```python
from build123d import *

# Parameters (mm, degrees)
STOCK_ACRYLIC_BAY_WALL_MASTER_1_START     = 163.456714755
STOCK_ACRYLIC_BAY_WALL_MASTER_1_OUTLINE_R = 2
STOCK_ACRYLIC_BAY_WALL_MASTER_1_DEPTH     = 5
SKETCH1_W                                 = 243.769145362
SKETCH1_H                                 = 5
BOSS_EXTRUDE1_DEPTH                       = 5
SKETCH2_W                                 = 25.2
SKETCH2_H                                 = 5
CUT_EXTRUDE1_DEPTH                        = 158.991773268
SKETCH3_R                                 = 1.6
CUT_EXTRUDE2_DEPTH                        = 158.991773268
SKETCH4_R                                 = 2
SKETCH4_W                                 = 27
SKETCH4_H                                 = 46.8
CUT_EXTRUDE3_DEPTH                        = 158.991773268
SKETCH5_R                                 = 22.5
SKETCH5_R_2                               = 1.6
CUT_EXTRUDE4_DEPTH                        = 158.991773268


# Read off the part's stored shape, not the designer's step: Stock-acrylic-bay-wall-master-1
with BuildPart() as part:
    # Stock-acrylic-bay-wall-master-1 outline → Stock-acrylic-bay-wall-master-1 (new body)
    with BuildSketch(Plane(origin=(0, 0, 0), x_dir=(0.866025403784438, 0, 0.500000000000001), z_dir=(0.500000000000001, 0, -0.866025403784438)).offset(STOCK_ACRYLIC_BAY_WALL_MASTER_1_START)):
        Polygon((-121.884572681, 15), (121.884572681, 15), (121.884572681, 89.75), (62.4, 89.75), (62.4, 95), (37.6, 95), (37.6, 89.75), (12.4, 89.75), (12.4, 95), (-12.4, 95), (-12.4, 89.75), (-37.6, 89.75), (-37.6, 95), (-62.4, 95), (-62.4, 89.75), (-121.884572681, 89.75), align=None)
        with Locations((-87.134572681, 35)):
            Circle(STOCK_ACRYLIC_BAY_WALL_MASTER_1_OUTLINE_R, mode=Mode.SUBTRACT)
        with Locations((87.134572681, 35)):
            Circle(STOCK_ACRYLIC_BAY_WALL_MASTER_1_OUTLINE_R, mode=Mode.SUBTRACT)
        with Locations((-112.134572681, 75)):
            Circle(STOCK_ACRYLIC_BAY_WALL_MASTER_1_OUTLINE_R, mode=Mode.SUBTRACT)
        with Locations((112.134572681, 75)):
            Circle(STOCK_ACRYLIC_BAY_WALL_MASTER_1_OUTLINE_R, mode=Mode.SUBTRACT)
    extrude(amount=STOCK_ACRYLIC_BAY_WALL_MASTER_1_DEPTH)

    # Sketch1 → Boss-Extrude1 (add)
    with BuildSketch(Plane(origin=(84.228357378, 0, -145.887794416), x_dir=(-0.8660254037844382, 0, -0.5000000000000009), z_dir=(0.5000000000000009, 0, -0.8660254037844382))):
        with Locations((0, -12.5)):
            Rectangle(SKETCH1_W, SKETCH1_H)
    extrude(amount=-BOSS_EXTRUDE1_DEPTH)

    # Sketch2 → Cut-Extrude1 (cut, through all)
    with BuildSketch(Plane(origin=(84.228357378, 0, -145.887794416), x_dir=(-0.8660254037844382, 0, -0.5000000000000009), z_dir=(0.5000000000000009, 0, -0.8660254037844382))):
        with Locations((-50, -17.5)):
            Rectangle(SKETCH2_W, SKETCH2_H)
        with Locations((0, -17.5)):
            Rectangle(SKETCH2_W, SKETCH2_H)
        with Locations((50, -17.5)):
            Rectangle(SKETCH2_W, SKETCH2_H)
    extrude(amount=-CUT_EXTRUDE1_DEPTH, mode=Mode.SUBTRACT)

    # Sketch3 → Cut-Extrude2 (cut, through all)
    with BuildSketch(Plane(origin=(84.228357378, 0, -145.887794416), x_dir=(-0.8660254037844382, 0, -0.5000000000000009), z_dir=(0.5000000000000009, 0, -0.8660254037844382))):
        with Locations((13.5, -40)):
            Circle(SKETCH3_R)
        with Locations((-13.5, -40)):
            Circle(SKETCH3_R)
        with Locations((15, -69.75)):
            Circle(SKETCH3_R)
        with Locations((-15, -69.75)):
            Circle(SKETCH3_R)
        with BuildLine():
            Line((10, -47), (10, -33))
            ThreePointArc((10, -33), (9.121320344, -30.878679656), (7, -30))
            Line((7, -30), (-7, -30))
            ThreePointArc((-7, -30), (-9.121320344, -30.878679656), (-10, -33))
            Line((-10, -33), (-10, -47))
            ThreePointArc((-10, -47), (-9.121320344, -49.121320344), (-7, -50))
            Line((-7, -50), (7, -50))
            ThreePointArc((7, -50), (9.121320344, -49.121320344), (10, -47))
        make_face()
        with BuildLine():
            Line((-6, -61.5), (6, -61.5))
            ThreePointArc((6, -61.5), (8.121320344, -62.378679656), (9, -64.5))
            Line((9, -64.5), (9, -75))
            ThreePointArc((9, -75), (8.121320344, -77.121320344), (6, -78))
            Line((6, -78), (-6, -78))
            ThreePointArc((-6, -78), (-8.121320344, -77.121320344), (-9, -75))
            Line((-9, -75), (-9, -64.5))
            ThreePointArc((-9, -64.5), (-8.121320344, -62.378679656), (-6, -61.5))
        make_face()
    extrude(amount=-CUT_EXTRUDE2_DEPTH, mode=Mode.SUBTRACT)

    # Sketch4 → Cut-Extrude3 (cut, through all)
    with BuildSketch(Plane(origin=(84.228357378, 0, -145.887794416), x_dir=(-0.8660254037844382, 0, -0.5000000000000009), z_dir=(0.5000000000000009, 0, -0.8660254037844382))):
        with Locations((69.1, -54.875)):
            Circle(SKETCH4_R)
        with Locations((30.9, -54.875)):
            Circle(SKETCH4_R)
        with Locations((50, -54.875)):
            Rectangle(SKETCH4_W, SKETCH4_H)
    extrude(amount=-CUT_EXTRUDE3_DEPTH, mode=Mode.SUBTRACT)

    # Sketch5 → Cut-Extrude4 (cut, through all)
    with BuildSketch(Plane(origin=(84.228357378, 0, -145.887794416), x_dir=(-0.8660254037844382, 0, -0.5000000000000009), z_dir=(0.5000000000000009, 0, -0.8660254037844382))):
        with Locations((-51.4, -54.875)):
            Circle(SKETCH5_R)
        with Locations((-71.4, -34.875)):
            Circle(SKETCH5_R_2)
        with Locations((-31.4, -34.875)):
            Circle(SKETCH5_R_2)
        with Locations((-31.4, -74.875)):
            Circle(SKETCH5_R_2)
        with Locations((-71.4, -74.875)):
            Circle(SKETCH5_R_2)
    extrude(amount=-CUT_EXTRUDE4_DEPTH, mode=Mode.SUBTRACT)


solid = part.part
```
For this review, take the finished solid that the model builds, in its own axes (mm). A direction names the side the tool comes from. Give positions to 0.01 mm unless a question says otherwise; leave off trailing zeros. Write each loop counter-clockwise with the first axis right and the second up, starting at its lowest first coordinate (ties: lowest second). Pieces come first, ordered by that corner, then holes. Notation, with made-up numbers: M 48,77.5 L 76,77.5 A14 ccw 76,88.5 Z; hole C -15.5,-33 d3. An arc over 180 degrees is marked long. Answer as a JSON object with one key per item and string values. Group by question number.
Item 1: Consider section C-C on z = -94. Write out the cut boundary in (x, y), plus the area to 4 significant figures.
Item 2: Draft analysis for pull direction Y (two halves, no side actions). For faces 4 (the flat face through (50.398, -92.338, -162.492)), 5 (the flat face through (40, -31.475, -169)), 6 (the flat face through (83, -15, -144)), 7 (the flat face through (84, -10, -143)), state which applies: +Y half, -Y half, draft (parallel to the pull), parting line (faces both ways), or undercut.
Item 3: For probe 1 along Y at (x, z) = (163, -99); probe 2 along Z at (x, y) = (83, -60); probe 3 along X at (y, z) = (-83, -201), list the stretches that pass through material, from the lowest coordinate up. Write a range as [from, to].
Item 4: Consider section B-B on x = 121. Count the separate pieces of the cut face and the enclosed holes in it, plus the area to 3 significant figures.
Item 5: Consider section A-A on y = -26. Write out the cut boundary in (x, z), plus the area to 3 significant figures.
Item 6: For pin 1 Ø1 at (x, y) = (95, -73) entering from -Z; pin 2 Ø6 at (y, z) = (-26.5, -152) entering from -X; pin 3 Ø3 at (x, y) = (93, -20) entering from -Z; pin 4 Ø8.5 at (x, z) = (86.5, -146.5) entering from +Y, all flat-tipped, find the tip position at first contact; note any pin that passes through.
Item 7: Tool access review of faces 1 (the cylindrical face through (54.6, -54.3, -160.2)), 2 (the flat face through (28.78, -17.54, -175.05)), 3 (the flat face through (137.209, -17.535, -112.453)): name each direction out of +Z, -Z, +X, -X, +Y, -Y from which nothing blocks a thin tool from reaching the whole face with its end or side.
Check result:
{
 "1": {"outline": "M 164.1,-89.75 L 174.1,-89.75 L 174.1,-10 L 164.1,-10 Z", "area": "797.5 mm^2"},
 "2": {"face 4": "draft", "face 5": "undercut", "face 6": "undercut", "face 7": "+Y half"},
 "3": {"probe 1": "y = [-89.75, -10]", "probe 2": "z = [-146.6, -140.82]", "probe 3": "x = [-21.23, -11.23]"},
 "4": {"separate pieces": "3", "enclosed holes": "0", "area": "217 mm^2"},
 "5": {"outline": "M -23.83,-202.5 L -21.33,-206.83 L 189.78,-84.95 L 187.28,-80.62 Z", "area": "1,220 mm^2"},
 "6": {"pin 1": "stops at z = -139.96", "pin 2": "stops at x = 58.45", "pin 3": "stops at z = -141.69", "pin 4": "stops at y = -10"},
 "7": {"face 1": "none", "face 2": "+Z, +X", "face 3": "-Z, -X"}
}
